Read the model definition and answer for the solid it produces. Units are mm, in the model's axes. A direction names the side the tool comes from. Give positions to 0.01 mm unless a question says otherwise; leave off trailing zeros. Order: outer loops, then holes, each group sorted by start corner. A loop starts at its lowest first (then second) coordinate and runs counter-clockwise, first axis right, second up. Notation, with made-up numbers: (-26.75, 51) - (6.25, 51) arc R24 ccw to (6.25, 75) - close; hole circle Ø5 at (83, 84). An arc over 180 degrees is marked (long way). Write item = value, one per line.
```python
from build123d import *

# Parameters (mm, degrees)
SKETCH_1_W             = 22
SKETCH_1_H             = 30
EXTRUDE_1_DEPTH        = 8
SKETCH_2_R             = 4.5
CUT_EXTRUDE_1_DEPTH    = 9
SKETCH_3_W             = 7
SKETCH_3_H             = 8
CUT_EXTRUDE_2_DEPTH    = 9
SKETCH_4_R             = 5.25
CUT_EXTRUDE_3_DEPTH    = 1
SKETCH_5_R             = 5.25
CUT_EXTRUDE_4_DEPTH    = 1
SKETCH_6_W             = 22
SKETCH_6_H             = 5
EXTRUDE_2_DEPTH        = 12
CUT_EXTRUDE_5_DEPTH    = 2.5
PATTERN_LINEAR_1_COUNT = 2
PATTERN_LINEAR_1_PITCH = 10
SKETCH_8_R             = 1.5
CUT_EXTRUDE_6_DEPTH    = 28.5
PATTERN_LINEAR_2_COUNT = 2
PATTERN_LINEAR_2_PITCH = 10
EXTRUDE_3_DEPTH        = 3
SKETCH_12_R            = 1.5
CUT_EXTRUDE_7_DEPTH    = 26
SKETCH_14_R            = 1.5
CUT_EXTRUDE_8_DEPTH    = 26
CUT_EXTRUDE_9_DEPTH    = 3
PATTERN_LINEAR_3_COUNT = 2
PATTERN_LINEAR_3_PITCH = 10
SKETCH_16_W            = 20
SKETCH_16_H            = 22
CUT_EXTRUDE_10_DEPTH   = 3


with BuildPart() as part:
    # 草图1 → 凸台-拉伸1 (new body)
    with BuildSketch(Plane(origin=(0, 0, 0), x_dir=(0, 0, -1), z_dir=(1, 0, 0))):
        Rectangle(SKETCH_1_W, SKETCH_1_H)
    extrude(amount=EXTRUDE_1_DEPTH)

    # 草图2 → 切除-拉伸1 (cut, through all)
    with BuildSketch(Plane.ZY):
        with Locations((0, 4)):
            Circle(SKETCH_2_R)
    extrude(amount=-CUT_EXTRUDE_1_DEPTH, mode=Mode.SUBTRACT)

    # 草图3 → 切除-拉伸2 (cut, through all)
    with BuildSketch(Plane.ZY):
        with Locations((7.5, -6)):
            Rectangle(SKETCH_3_W, SKETCH_3_H)
    extrude(amount=-CUT_EXTRUDE_2_DEPTH, mode=Mode.SUBTRACT)

    # 草图4 → 切除-拉伸3 (cut)
    with BuildSketch(Plane.ZY):
        with Locations((0, 4)):
            Circle(SKETCH_4_R)
    extrude(amount=-CUT_EXTRUDE_3_DEPTH, mode=Mode.SUBTRACT)

    # 草图5 → 切除-拉伸4 (cut)
    with BuildSketch(Plane(origin=(8, 0, 0), x_dir=(0, 0, -1), z_dir=(1, 0, 0))):
        with Locations((0, 4)):
            Circle(SKETCH_5_R)
    extrude(amount=-CUT_EXTRUDE_4_DEPTH, mode=Mode.SUBTRACT)

    # 草图6 → 凸台-拉伸2 (add)
    with BuildSketch(Plane(origin=(8, 0, 0), x_dir=(0, 0, -1), z_dir=(1, 0, 0))):
        with Locations((0, -12.5)):
            Rectangle(SKETCH_6_W, SKETCH_6_H)
    extrude(amount=EXTRUDE_2_DEPTH)

    # 草图7 → 切除-拉伸5 (cut)
    with BuildSketch(Plane.XZ.offset(15)):
        Polygon((9.8, -5), (11.4, -7.771281292), (14.6, -7.771281292), (16.2, -5), (14.6, -2.228718708), (11.4, -2.228718708), align=None)
    cut_extrude_5 = extrude(amount=-CUT_EXTRUDE_5_DEPTH, mode=Mode.SUBTRACT)

    # 阵列(线性)1: 切除-拉伸5 ×2
    with Locations(*[(0, 0, i * PATTERN_LINEAR_1_PITCH) for i in range(1, PATTERN_LINEAR_1_COUNT)]):
        add(cut_extrude_5, mode=Mode.SUBTRACT)

    # 草图8 → 切除-拉伸6 (cut, through all)
    with BuildSketch(Plane.XZ.offset(12.5)):
        with Locations((13, 5)):
            Circle(SKETCH_8_R)
    cut_extrude_6 = extrude(amount=-CUT_EXTRUDE_6_DEPTH, mode=Mode.SUBTRACT)

    # 阵列(线性)2: 切除-拉伸6 ×2
    with Locations(*[(0, 0, -i * PATTERN_LINEAR_2_PITCH) for i in range(1, PATTERN_LINEAR_2_COUNT)]):
        add(cut_extrude_6, mode=Mode.SUBTRACT)

    # 草图10 → 凸台-拉伸3 (add)
    with BuildSketch(Plane(origin=(0, -10, 0), x_dir=(1, 0, 0), z_dir=(0, 1, 0))):
        Polygon((0, -4), (8, -4), (8, 11), (20, 11), (20, -11), (0, -11), align=None)
    extrude(amount=EXTRUDE_3_DEPTH)

    # 草图12 → 切除-拉伸7 (cut, through all)
    with BuildSketch(Plane.XZ.offset(10)):
        with Locations((13, 5)):
            Circle(SKETCH_12_R)
    extrude(amount=-CUT_EXTRUDE_7_DEPTH, mode=Mode.SUBTRACT)

    # 草图14 → 切除-拉伸8 (cut, through all)
    with BuildSketch(Plane.XZ.offset(10)):
        with Locations((13, -5)):
            Circle(SKETCH_14_R)
    extrude(amount=-CUT_EXTRUDE_8_DEPTH, mode=Mode.SUBTRACT)

    # 草图15 → 切除-拉伸9 (cut)
    with BuildSketch(Plane.XZ.offset(12.5)):
        Polygon((16.2, 5), (14.6, 7.771281292), (11.4, 7.771281292), (9.8, 5), (11.4, 2.228718708), (14.6, 2.228718708), align=None)
    cut_extrude_9 = extrude(amount=-CUT_EXTRUDE_9_DEPTH, mode=Mode.SUBTRACT)

    # 阵列(线性)3: 切除-拉伸9 ×2
    with Locations(*[(0, 0, -i * PATTERN_LINEAR_3_PITCH) for i in range(1, PATTERN_LINEAR_3_COUNT)]):
        add(cut_extrude_9, mode=Mode.SUBTRACT)

    # 草图16 → 切除-拉伸10 (cut)
    with BuildSketch(Plane.XZ.offset(15)):
        with Locations((10, 0)):
            Rectangle(SKETCH_16_W, SKETCH_16_H)
    extrude(amount=-CUT_EXTRUDE_10_DEPTH, mode=Mode.SUBTRACT)


solid = part.part
```
1. For faces 1 (the face through (10.59, -10.77, -6.37)), 2 (the face through (12, -7, 2)), 3 (the face through (11.5, -8.27, -4.93)), determine the directions among +Z, -Z, +X, -X, +Y, -Y from which every point of the face is accessible in a straight line to the end or side of a thin tool.
Recorded:
face_1 = -Y
face_2 = +Z, +X
face_3 = +Y, -Y
2. Section A-A (z = 0) is taken. Determine the outline of the cut face in (x, y).
Recorded:
outline = (0, -12) - (20, -12) - (20, -7) - (8, -7) - (8, -1.25) - (7, -1.25) - (7, -0.5) - (1, -0.5) - (1, -1.25) - (0, -1.25) - close; (0, 9.25) - (1, 9.25) - (1, 8.5) - (7, 8.5) - (7, 9.25) - (8, 9.25) - (8, 15) - (0, 15) - close
3. Determine the mould class of faces 4 (the face through (15.41, -10.77, -3.63)), 5 (the face through (4, -2, 7)), 6 (the face through (4, 6, 11)) for opening direction Z: +Z half, -Z half, draft (parallel to the pull), parting line (faces both ways), or undercut.
Recorded:
face_4 = undercut
face_5 = draft
face_6 = +Z half
4. Section B-B (y = 4) is taken. Determine the outline of the cut face in (x, z), and give its area (3 significant figures).
Recorded:
outline = (0, -11) - (8, -11) - (8, -5.25) - (7, -5.25) - (7, -4.5) - (1, -4.5) - (1, -5.25) - (0, -5.25) - close; (0, 5.25) - (1, 5.25) - (1, 4.5) - (7, 4.5) - (7, 5.25) - (8, 5.25) - (8, 11) - (0, 11) - close
area = 101 mm^2
5. Section C-C (x = 5.75) is taken. Determine the outline of the cut face in (y, z), and give its area (3 significant figures).
Recorded:
outline = (-12, -11) - (15, -11) - (15, 11) - (-2, 11) - (-2, 4) - (-7, 4) - (-7, 11) - (-12, 11) - close; hole circle Ø9 at (4, 0)
area = 495 mm^2
6. Section D-D (z = 9) is taken. Determine the outline of the cut face in (x, y).
Recorded:
outline = (0, -12) - (20, -12) - (20, -7) - (0, -7) - close; (0, -2) - (8, -2) - (8, 15) - (0, 15) - close
7. Straight lines are drawn through the part: L1, parallel to Z at x = 13, y = -7.6; L2, parallel to Y at x = 3.5, z = 0; L3, parallel to X at y = 14.25, z = 6.5. For each, find the intervals that lie inside material, in ascending order. Write a range as [from, to].
Recorded:
L1 = [-11, -6.5], [-3.5, 3.5], [6.5, 11]
L2 = [-12, -0.5], [8.5, 15]
L3 = [0, 8]
8. Flat-ended cylindrical pins translate along their axes: pin 1 (8.5 mm diameter, centred on y = 2.5, z = 0.5, fed in from +X); pin 2 (2 mm diameter, centred on x = 8, y = -3.5, fed in from +Z); pin 3 (2 mm diameter, centred on y = 2.5, z = 3.5, fed in from -X); pin 4 (2.5 mm diameter, centred on x = 13, z = 5, fed in from +Y). Find the tip coordinate at first contact, or state that the pin passes through.
Recorded:
pin_1 = 8
pin_2 = 4
pin_3 = 1
pin_4 = through
